Here's how the part is built. I have some questions about the finished solid (model axes, mm). A direction names the side the tool comes from. Round coordinates to 2 decimals unless told otherwise and drop trailing zeros. Loops run counter-clockwise (first coordinate to the right, second up) from the corner with the lowest first, then second, coordinate; pieces in that order, holes last. Notation, with made-up numbers: M 50,29 L 88,29 A28 cw 88,54 Z; hole C 62.25,69 d5. An arc over 180 degrees is marked long. Answer as a JSON object with one key per item and string values.
from build123d import *

# Parameters (mm, degrees)
SKETCH1_R           = 29
SKETCH1_R_2         = 2.5
BOSS_EXTRUDE1_DEPTH = 2
SKETCH2_R           = 26
SKETCH2_R_2         = 25
BOSS_EXTRUDE2_DEPTH = 3
BOSS_EXTRUDE3_DEPTH = 2
SKETCH4_W           = 2
SKETCH4_H           = 10
BOSS_EXTRUDE4_DEPTH = 10
FILLET1_R           = 2
SKETCH5_R           = 2.5
CUT_EXTRUDE1_DEPTH  = 56.686623169


with BuildPart() as part:
    # Sketch1 → Boss-Extrude1 (new body)
    with BuildSketch(Plane.XY):
        Circle(SKETCH1_R)
        Circle(SKETCH1_R_2, mode=Mode.SUBTRACT)
    extrude(amount=BOSS_EXTRUDE1_DEPTH)

    # Sketch2 → Boss-Extrude2 (add)
    with BuildSketch(Plane.XY.offset(2)):
        Circle(SKETCH2_R)
        Circle(SKETCH2_R_2, mode=Mode.SUBTRACT)
    extrude(amount=BOSS_EXTRUDE2_DEPTH)

    # Sketch3 → Boss-Extrude3 (add)
    with BuildSketch(Plane(origin=(0, 0, 0), x_dir=(-1, 0, 0), z_dir=(0, 0, -1))):
        with BuildLine():
            Line((-13.75, 7.5), (-13.75, -7.5))
            ThreePointArc((-13.75, -7.5), (-16, -9.75), (-18.25, -7.5))
            Line((-18.25, -7.5), (-18.25, 7.5))
            ThreePointArc((-18.25, 7.5), (-16, 9.75), (-13.75, 7.5))
        make_face()
        with BuildLine():
            Line((18.25, 7.5), (18.25, -7.5))
            ThreePointArc((18.25, -7.5), (16, -9.75), (13.75, -7.5))
            Line((13.75, -7.5), (13.75, 7.5))
            ThreePointArc((13.75, 7.5), (16, 9.75), (18.25, 7.5))
        make_face()
    extrude(amount=BOSS_EXTRUDE3_DEPTH)

    # Sketch4 → Boss-Extrude4 (add)
    with BuildSketch(Plane(origin=(0, 0, -2), x_dir=(-1, 0, 0), z_dir=(0, 0, -1))):
        with Locations((-16, 0.07539605)):
            Rectangle(SKETCH4_W, SKETCH4_H)
        with Locations((16, 0.07539605)):
            Rectangle(SKETCH4_W, SKETCH4_H)
    extrude(amount=BOSS_EXTRUDE4_DEPTH)

    # Fillet1
    fillet1_edges = [part.edges().sort_by_distance(p)[0] for p in [
        (16, 5.07539605, -12),
        (16, -4.92460395, -12),
        (-16, 5.07539605, -12),
        (-16, -4.92460395, -12),
    ]]
    fillet(fillet1_edges, radius=FILLET1_R)

    # Sketch5 → Cut-Extrude1 (cut, through all)
    with BuildSketch(Plane.ZY.offset(17)):
        with Locations(Location((-8, 0, 0), (0, 0, 270))):
            Circle(SKETCH5_R)
    extrude(amount=-CUT_EXTRUDE1_DEPTH, mode=Mode.SUBTRACT)


solid = part.part
Item 1: I want a section at C-C on z = -3.25. List the corners of the cut face in (x, y) for me.
Solution:
{"outline": "M -17,-4.92 L -15,-4.92 L -15,5.08 L -17,5.08 Z; M 15,-4.92 L 17,-4.92 L 17,5.08 L 15,5.08 Z"}
Item 2: We'd pull the mould along X, two halves only. Please class faces 4 (the face through (-15, 0, -5)), 5 (the face through (14, 0, -2)), 6 (the face through (-18.25, 0, -1)), 7 (the face through (-16.01, 0.54, -10.44)): +X half, -X half, draft (parallel to the pull), parting line (faces both ways), or undercut.
Solution:
{"face 4": "undercut", "face 5": "undercut", "face 6": "-X half", "face 7": "draft"}
Item 3: I want a section at D-D on y = 0. Count the separate pieces of the cut face and the enclosed holes in it, plus the area to 3 significant figures.
Solution:
{"separate pieces": "4", "enclosed holes": "0", "area": "150 mm2"}
Item 4: For faces 1 (the face through (-16, -4.925, -6)), 2 (the face through (23.846, 7.509, 3.479)), 3 (the face through (15, 0, -5)), which set-ups out of +Z, -Z, +X, -X, +Y, -Y let a thin tool reach every point of the face, with its end or its side?
Solution:
{"face 1": "-Z, +X, -X, -Y", "face 2": "+Z", "face 3": "-Z, +Y, -Y"}
Item 5: I want a section at B-B on z = -8. List the corners of the cut face in (x, y) for me.
Solution:
{"outline": "M -17,-4.92 L -15,-4.92 L -15,-2.5 L -17,-2.5 Z; M -17,2.5 L -15,2.5 L -15,5.08 L -17,5.08 Z; M 15,-4.92 L 17,-4.92 L 17,-2.5 L 15,-2.5 Z; M 15,2.5 L 17,2.5 L 17,5.08 L 15,5.08 Z"}
Item 6: For P1, Ø3, axis at y = -6, z = -5.5, coming from the -X side; P2, Ø12, axis at x = -2.5, y = -8, coming from the +Z side; P3, Ø2, axis at x = -16, z = -5.5, coming from the +Y side, each with a flat end and sliding along its axis, tell me the tip position at first contact or that it passes through.
Solution:
{"P1": "stops at x = -17", "P2": "stops at z = 2", "P3": "stops at y = 5.08"}
Item 7: If I drill on L1, parallel to X at y = 0.5, z = -3.25; L2, parallel to Y at x = 0, z = 1.15; L3, parallel to Z at x = 19, y = 5, over which ranges is the centre line in solid material (lowest first)? Write a range as from..to.
Solution:
{"L1": "x = -17..-15, 15..17", "L2": "y = -29..-2.5, 2.5..29", "L3": "z = 0..2"}
Item 8: I want a section at A-A on x = 0. List the corners of the cut face in (y, z) for me.
Solution:
{"outline": "M -29,0 L -2.5,0 L -2.5,2 L -25,2 L -25,5 L -26,5 L -26,2 L -29,2 Z; M 2.5,0 L 29,0 L 29,2 L 26,2 L 26,5 L 25,5 L 25,2 L 2.5,2 Z"}
